from build123d import *

# Parameters (mm, degrees)
F1_DEPTH = 177.8
F2_W     = 50.8
F2_H     = 25.4
F3_DEPTH = 25.4
F4_W     = 50.8
F4_H     = 25.4
F5_DEPTH = 25.4
F7_DEPTH = 101.6


with BuildPart() as f1:
    # F0 (on Front) → F1 (new body)
    with BuildSketch(Plane.XZ):
        Polygon((-99.25165, 100.57334), (-99.25165, -26.42666), (103.94835, -26.42666), (103.94835, 24.37334), (-48.45165, 24.37334), (-48.45165, 100.57334), align=None)
    extrude(amount=F1_DEPTH)

    # F2 (on face) → F3 (join)
    with BuildSketch(Plane.XY.offset(100.57334)):
        with Locations((-73.85165, -165.1)):
            Rectangle(F2_W, F2_H)
    extrude(amount=F3_DEPTH)

    # F4 (on face) → F5 (join)
    with BuildSketch(Plane.XY.offset(100.57334)):
        with Locations((-73.85165, -12.7)):
            Rectangle(F4_W, F4_H)
    extrude(amount=F5_DEPTH)

    # F6 (on face) → F7 (cut)
    with BuildSketch(Plane.YZ.offset(103.94835)):
        Polygon((-127, 24.37334), (-127, -1.02666), (-127, -26.42666), (-50.8, -26.42666), (-50.8, 0), (-50.8, 24.37334), align=None)
    extrude(amount=-F7_DEPTH, mode=Mode.SUBTRACT)


solid = f1.part
Input: part model. Units: mm. Frame: model coordinates. A direction names the side the tool comes from. Give positions to 0.01 mm unless a question says otherwise; leave off trailing zeros. Loops run counter-clockwise (first coordinate to the right, second up) from the corner with the lowest first, then second, coordinate; pieces in that order, holes last. Notation, with made-up numbers: M 0.25,-11.5 L 18.25,-11.5 A16 cw 18.25,9.5 Z; hole C 23.25,40.25 d7. An arc over 180 degrees is marked long. Use one line per item in the form item = value.
1. Section query D-D, the plane x = -25. Return the cut outline in (y, z), and give its area (3 significant figures).
Numbers:
outline = M -177.8,-26.43 L 0,-26.43 L 0,24.37 L -177.8,24.37 Z
area = 9,030 mm²
2. Reachability of faces 1 (the face through (1, -88, -26.427)), 2 (the face through (-5, -88, 24.373)), 3 (the face through (-73, -88, 100.573)), 4 (the face through (54, -50.8, -1)), 5 (the face through (103.948, -152, -1)) from +Z, -Z, +X, -X, +Y, -Y: full face, straight path, thin tool, end or side. Return the list, or none.
Numbers:
face_1 = -Z, +X, -X, +Y, -Y
face_2 = +Z, +X, +Y, -Y
face_3 = +Z, +X, -X
face_4 = +Z, -Z, +X
face_5 = +Z, -Z, +X, +Y, -Y
3. First-contact query: pin 1 (6 mm diameter, centred on x = -14.5, y = -49.5, fed in from +Z); pin 2 (15 mm diameter, centred on y = -96.5, z = -11.5, fed in from +X). Flat tips, straight axial feed; report the tip coordinate or a pass-through.
Numbers:
pin_1 = 24.37
pin_2 = 2.35
4. Section query B-B, the plane z = 12.5. Return the cut outline in (x, y).
Numbers:
outline = M -99.25,-177.8 L 103.95,-177.8 L 103.95,-127 L 2.35,-127 L 2.35,-50.8 L 103.95,-50.8 L 103.95,0 L -99.25,0 Z
5. Section query A-A, the plane x = 44. Return the cut outline in (y, z), and give its area (3 significant figures).
Numbers:
outline = M -177.8,-26.43 L -127,-26.43 L -127,24.37 L -177.8,24.37 Z; M -50.8,-26.43 L 0,-26.43 L 0,24.37 L -50.8,24.37 Z
area = 5,160 mm²
6. Line query: L1, parallel to X at y = -149, z = 67.5; L2, parallel to Z at x = 59.5, y = -129.5; L3, parallel to Z at x = -60, y = -39. Output: solid intervals per line, ascending.
Numbers:
L1 = -99.25 to -48.45
L2 = -26.43 to 24.37
L3 = -26.43 to 100.57
7. Section query C-C, the plane y = -157.5. Return the cut outline in (x, z), and give its area (3 significant figures).
Numbers:
outline = M -99.25,-26.43 L 103.95,-26.43 L 103.95,24.37 L -48.45,24.37 L -48.45,125.97 L -99.25,125.97 Z
area = 15,500 mm²
8. Pull-direction query (Y, two-part tool) for faces 6 (the face through (-74, -25.4, 113)), 7 (the face through (-48.452, -90, 63)), 8 (the face through (-22, -177.8, 15)); classes: released by +Y, released by -Y, zero draft, split by the parting line, or undercut.
Numbers:
face_6 = undercut
face_7 = zero draft
face_8 = released by -Y
